```python
from build123d import *

# Parameters (mm, degrees)
F1_DEPTH = 4
F2_W     = 27
F2_H     = 31
F3_DEPTH = 28
F4_R     = 2
F5_R     = 5
F6_R     = 1.5
F7_DEPTH = 25
F8_SIZE  = 6
F9_R     = 5
F10_R    = 5


with BuildPart() as f1:
    # F0 (on Front) → F1 (new body)
    with BuildSketch(Plane.XZ):
        Polygon((-13, -17), (13, -17), (22.5, 0), (13, 17), (-13, 17), (-22.5, 0), align=None)
    extrude(amount=F1_DEPTH)

    # F2 (on face) → F3 (join)
    with BuildSketch(Plane(origin=(0, 0, 0), x_dir=(-1, 0, 0), z_dir=(0, 1, 0))):
        Rectangle(F2_W, F2_H)
    extrude(amount=F3_DEPTH)

    # F4
    f4_edges = [f1.edges().sort_by_distance(p)[0] for p in [
        (-13.5, 14, 15.5),
        (13.5, 14, 15.5),
    ]]
    fillet(f4_edges, radius=F4_R)

    # F5
    f5_edges = [f1.edges().sort_by_distance(p)[0] for p in [
        (-22.5, -2, 0),
        (22.5, -2, 0),
    ]]
    fillet(f5_edges, radius=F5_R)

    # F6 (on face) → F7 (cut)
    with BuildSketch(Plane.XZ.offset(4)):
        with Locations((-18, 0)):
            Circle(F6_R)
        with Locations((18, 0)):
            Circle(F6_R)
    extrude(amount=-F7_DEPTH, mode=Mode.SUBTRACT)

    # F8
    f8_edges = [f1.edges().sort_by_distance(p)[0] for p in [
        (13.5, 14, -15.5),
        (-13.5, 14, -15.5),
    ]]
    chamfer(f8_edges, length=F8_SIZE)

    # F9
    f9_edges = [f1.edges().sort_by_distance(p)[0] for p in [
        (13, -2, 17),
        (-13, -2, 17),
        (13, -2, -17),
        (-13, -2, -17),
    ]]
    fillet(f9_edges, radius=F9_R)

    # F10
    f10_edges = [f1.edges().sort_by_distance(p)[0] for p in [
        (-13.5, 14, -9.5),
        (-7.5, 14, -15.5),
        (7.5, 14, -15.5),
        (13.5, 14, -9.5),
    ]]
    fillet(f10_edges, radius=F10_R)


solid = f1.part
```
Check sheet for the modelled part. Datum: model origin and axes. Units: mm. A direction names the side the tool comes from. Give positions to 0.01 mm unless a question says otherwise; leave off trailing zeros. Order: outer loops, then holes, each group sorted by start corner. A loop starts at its lowest first (then second) coordinate and runs counter-clockwise, first axis right, second up. Notation, with made-up numbers: (-3.5, -18.75) -> (0.5, -18.75) arc R18 cw to (0.5, 11.25) -> close; hole circle Ø11 at (46.25, 54.25). An arc over 180 degrees is marked (long way). Return JSON: item names as keys, results as strings.
1. Material ranges on probe 1 along Z at (x, y) = (18, -2.75); probe 2 along X at (y, z) = (2.5, 9.5); probe 3 along X at (y, z) = (22, -11.5), recorded low to high. Write a range as [from, to].
From the geometry:
{"probe 1": "[-8.05, -1.5], [1.5, 8.05]", "probe 2": "[-13.5, 13.5]", "probe 3": "[-11.5, 11.5]"}
2. Set-up check for faces 1 (the cylindrical face through (-12.9, 14.2, 14.93)), 2 (the cylindrical face through (7.37, 14.2, -15.11)), 3 (the flat face through (-13.5, 14, 3)): record each of +Z, -Z, +X, -X, +Y, -Y from which the full face is reachable in a straight line by a thin tool's end or side.
From the geometry:
{"face 1": "+Z, -X, +Y", "face 2": "-Z, +X, +Y", "face 3": "+Z, -Z, -X, +Y"}
3. Cross-section at C-C, the plane x = -18. Record the cut outline in (y, z), plus the area to 3 significant figures.
From the geometry:
{"outline": "(-4, -8.05) -> (0, -8.05) -> (0, -1.5) -> (-4, -1.5) -> close; (-4, 1.5) -> (0, 1.5) -> (0, 8.05) -> (-4, 8.05) -> close", "area": "52.4 mm^2"}
4. Cross-section at A-A, the plane z = 0. Record the cut outline in (x, y).
From the geometry:
{"outline": "(-21.77, -4) -> (-19.5, -4) -> (-19.5, 0) -> (-21.77, 0) -> close; (-16.5, -4) -> (16.5, -4) -> (16.5, 0) -> (13.5, 0) -> (13.5, 28) -> (-13.5, 28) -> (-13.5, 0) -> (-16.5, 0) -> close; (19.5, -4) -> (21.77, -4) -> (21.77, 0) -> (19.5, 0) -> close"}
5. Cross-section at B-B, the plane y = 12.5. Record the cut outline in (x, z), plus the area to 3 significant figures.
From the geometry:
{"outline": "(-13.5, -7.43) arc R5 ccw to (-12.04, -10.96) -> (-8.96, -14.04) arc R5 ccw to (-5.43, -15.5) -> (5.43, -15.5) arc R5 ccw to (8.96, -14.04) -> (12.04, -10.96) arc R5 ccw to (13.5, -7.43) -> (13.5, 13.5) arc R2 ccw to (11.5, 15.5) -> (-11.5, 15.5) arc R2 ccw to (-13.5, 13.5) -> close", "area": "797 mm^2"}
6. Mould release check, pull along Z, two halves, no side actions. Record for faces 4 (the cylindrical face through (21.772, -2.028, -0.036)), 5 (the cylindrical face through (-7.32, 14.2, -15.13)), 6 (the cylindrical face through (-19.5, -2.03, 0.07)): +Z half, -Z half, draft (parallel to the pull), parting line (faces both ways), or undercut.
From the geometry:
{"face 4": "parting line", "face 5": "-Z half", "face 6": "undercut"}
7. Go/stop test with flat-tipped pins: P1, Ø3, axis at x = 12, y = 7, coming from the -Z side; P2, Ø5, axis at y = 7, z = -8, coming from the -X side; P3, Ø3.5, axis at x = -1.5, y = 13, coming from the -Z side. Record where each tip stops, or that it passes through.
From the geometry:
{"P1": "z = -12.5", "P2": "x = -13.5", "P3": "z = -15.5"}
8. Cross-section at D-D, the plane z = 10. Record the cut outline in (x, y), plus the area to 3 significant figures.
From the geometry:
{"outline": "(-16.91, -4) -> (16.91, -4) -> (16.91, 0) -> (13.5, 0) -> (13.5, 28) -> (-13.5, 28) -> (-13.5, 0) -> (-16.91, 0) -> close", "area": "891 mm^2"}
